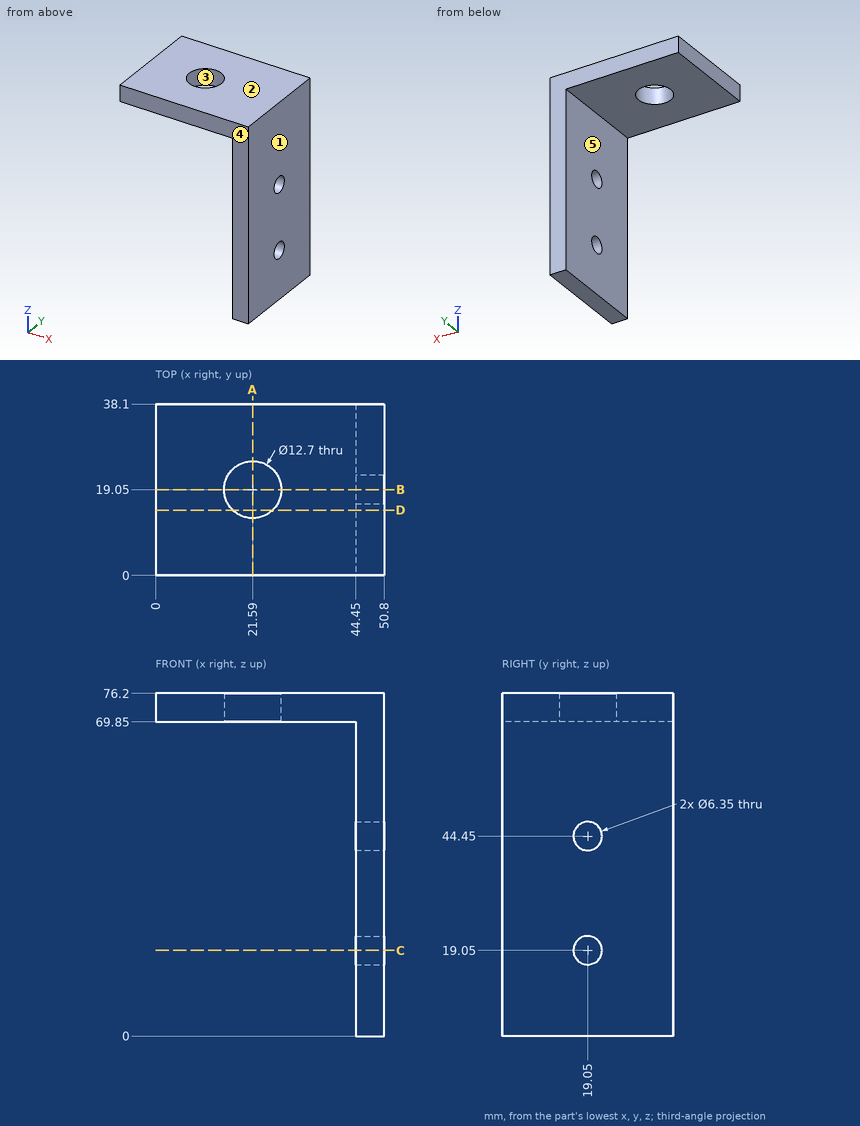
Input: dimensioned drawing with shaded views. Units: mm. Origin: part minimum x, y, z. A direction names the side the tool comes from. Give positions to 0.01 mm unless a question says otherwise; leave off trailing zeros. Write each loop counter-clockwise with the first axis right and the second up, starting at its lowest first coordinate (ties: lowest second). Pieces come first, ordered by that corner, then holes. Notation, with made-up numbers: (46, 37.5) -> (76, 37.5) arc R16 cw to (76, 51.5) -> close; hole circle Ø6 at (43.5, -22.5). An arc over 180 degrees is marked (long way). Return JSON: item names as keys, results as strings. Group by question number.
1. Access query for the marked faces 4 and 5. Directions: +Z, -Z, +X, -X, +Y, -Y. A direction counts if a zero-diameter tool reaches every point of the face in a straight line with its end or side. Return the directions, or none.
2. Section C-C, the plane z = 19.05. Output: boundary loops of the cut face in (x, y) (3 decimals), then the cut area to 3 significant figures.
3. Section A-A, the plane x = 21.59. Output: boundary loops of the cut face in (y, z).
4. Section B-B, the plane y = 19.05. Output: boundary loops of the cut face in (x, z) (3 decimals), then the cut area to 3 significant figures.
5. Material intervals for line 1 (Z direction, x = 48.5, y = 19.05) (3 decimals); line 2 (Y direction, x = 46, z = 19); line 3 (X direction, y = 2, z = 23.5), sorted ascending. Write a range as from..to.
6. Pin query (flat end, axial travel): pin 1 Ø12 at (y, z) = (20.5, 38.5) entering from -X; pin 2 Ø8 at (x, y) = (8.5, 12) entering from -Z. Return the tip coordinate at first contact, or that it passes through.
7. Mould query, pull axis X, two halves, no side actions, for the marked faces 1, 2 and 3. Classes: +X half, -X half, draft (parallel to the pull), parting line (faces both ways), or undercut.
8. Section D-D, the plane y = 14.5. Output: boundary loops of the cut face in (x, z), then the cut area to 3 significant figures.
Determined:
{
 "1": {"face 4": "+Z, -Z, +X, -X, -Y", "face 5": "-Z, -X, +Y, -Y"},
 "2": {"outline": "(44.45, 0) -> (50.8, 0) -> (50.8, 15.875) -> (44.45, 15.875) -> close; (44.45, 22.225) -> (50.8, 22.225) -> (50.8, 38.1) -> (44.45, 38.1) -> close", "area": "202 mm2"},
 "3": {"outline": "(0, 69.85) -> (12.7, 69.85) -> (12.7, 76.2) -> (0, 76.2) -> close; (25.4, 69.85) -> (38.1, 69.85) -> (38.1, 76.2) -> (25.4, 76.2) -> close"},
 "4": {"outline": "(0, 69.85) -> (15.24, 69.85) -> (15.24, 76.2) -> (0, 76.2) -> close; (27.94, 69.85) -> (44.45, 69.85) -> (44.45, 47.625) -> (50.8, 47.625) -> (50.8, 76.2) -> (27.94, 76.2) -> close; (44.45, 0) -> (50.8, 0) -> (50.8, 15.875) -> (44.45, 15.875) -> close; (44.45, 22.225) -> (50.8, 22.225) -> (50.8, 41.275) -> (44.45, 41.275) -> close", "area": "605 mm2"},
 "5": {"line 1": "z = 0..15.875, 22.225..41.275, 47.625..76.2", "line 2": "y = 0..15.88, 22.22..38.1", "line 3": "x = 44.45..50.8"},
 "6": {"pin 1": "stops at x = 44.45", "pin 2": "stops at z = 69.85"},
 "7": {"face 1": "+X half", "face 2": "draft", "face 3": "undercut"},
 "8": {"outline": "(0, 69.85) -> (17.16, 69.85) -> (17.16, 76.2) -> (0, 76.2) -> close; (26.02, 69.85) -> (44.45, 69.85) -> (44.45, 0) -> (50.8, 0) -> (50.8, 76.2) -> (26.02, 76.2) -> close", "area": "710 mm2"}
}
